Model file for the job. Use its own axes, mm. A direction names the side the tool comes from. Give positions to 0.01 mm unless a question says otherwise; leave off trailing zeros. Loops run counter-clockwise (first coordinate to the right, second up) from the corner with the lowest first, then second, coordinate; pieces in that order, holes last. Notation, with made-up numbers: M -15.5,37.25 L 17.5,37.25 A30 ccw 17.5,59.25 Z; hole C 17,-1.5 d11. An arc over 180 degrees is marked long. Use CSV: the item, a comma, the result in double quotes. Start each with the question number.
(1) Slice it at A-A on y = -2.75. List the corners of the cut face in (x, z), and give its area (3 significant figures).
(2) Two-plate mould, pull along Y, no slides. Class faces 1 (the face through (-1, 0, 25)), 2 (the face through (0, 0, 0)), 3 (the face through (-1, 15, 0)): pulls with the +Y half, pulls with the -Y half, needs draft (parallel to the pull), parting line crosses it, or undercut.
(3) Slice it at B-B on x = 0. List the corners of the cut face in (y, z), and give its area (3 significant figures).
(4) Flat gauge pin, fed straight in: P1, Ø8, axis at x = -3.5, z = -2, coming from the -Y side. Where does the tip first touch, or does it go through?
(5) Slice it at C-C on z = 0. List the corners of the cut face in (x, y), and give its area (3 significant figures).
(6) Tool access for faces 4 (the face through (-50, 0, 0)), 5 (the face through (7.62, -7.4, -3.16)): list every direction of +Z, -Z, +X, -X, +Y, -Y with a clear straight run to the whole face (end or side of a thin tool).
(7) Wall check: line 1 along Z through (x, y) = (0, -5.25); line 2 along X through (y, z) = (-7.5, 0); line 3 along Z through (x, y) = (-1.5, -8). Give the ranges that are in metal, low to high. Write a range as from..to.
```python
from build123d import *

# Parameters (mm, degrees)
F0_W      = 100
F0_H      = 50
F1_DEPTH  = 15
F2_R      = 8.25
F1_FACE_W = 100
F1_FACE_H = 50
F3_DEPTH  = 20


with BuildPart() as f1:
    # F0 (on Front) → F1 (new body, symmetric)
    with BuildSketch(Plane.XZ):
        Rectangle(F0_W, F0_H)
    extrude(amount=F1_DEPTH, both=True)

    # F2 (on Front) + F1_face (on face) → F3 (cut)
    with BuildSketch(Plane.XZ):
        Circle(F2_R)
    with BuildSketch(Plane.XZ.offset(15)):
        Rectangle(F1_FACE_W, F1_FACE_H)
    extrude(amount=F3_DEPTH, mode=Mode.SUBTRACT)


solid = f1.part
```
Reply:
1,outline,"M -50,-25 L 50,-25 L 50,25 L -50,25 Z; hole C 0,0 d16.5"
1,area,"4,790 mm^2"
2,face 1,"needs draft"
2,face 2,"pulls with the -Y half"
2,face 3,"pulls with the +Y half"
3,outline,"M -15,-25 L 15,-25 L 15,25 L -15,25 L -15,8.25 L 0,8.25 L 0,-8.25 L -15,-8.25 Z"
3,area,"1,250 mm^2"
4,P1,"stops at y = 0"
5,outline,"M -50,-15 L -8.25,-15 L -8.25,0 L 8.25,0 L 8.25,-15 L 50,-15 L 50,15 L -50,15 Z"
5,area,"2,750 mm^2"
6,face 4,"+Z, -Z, -X, +Y, -Y"
6,face 5,"-Y"
7,line 1,"z = -25..-8.25, 8.25..25"
7,line 2,"x = -50..-8.25, 8.25..50"
7,line 3,"z = -25..-8.11, 8.11..25"
